The drawing under review shows one solid part. Ordinate dimensions are in mm from its lowest x, y, z. Coordinates: 2 decimals unless noted, no trailing zeros. Order: outer loops, then holes, each group sorted by start corner. A loop starts at its lowest first (then second) coordinate and runs counter-clockwise, first axis right, second up. Notation, with made-up numbers: M 46,46 L 82,46 A6 cw 82,53 Z; hole C 50,-4 d11. An arc over 180 degrees is marked long. Answer as a JSON object with one key per item and string values.
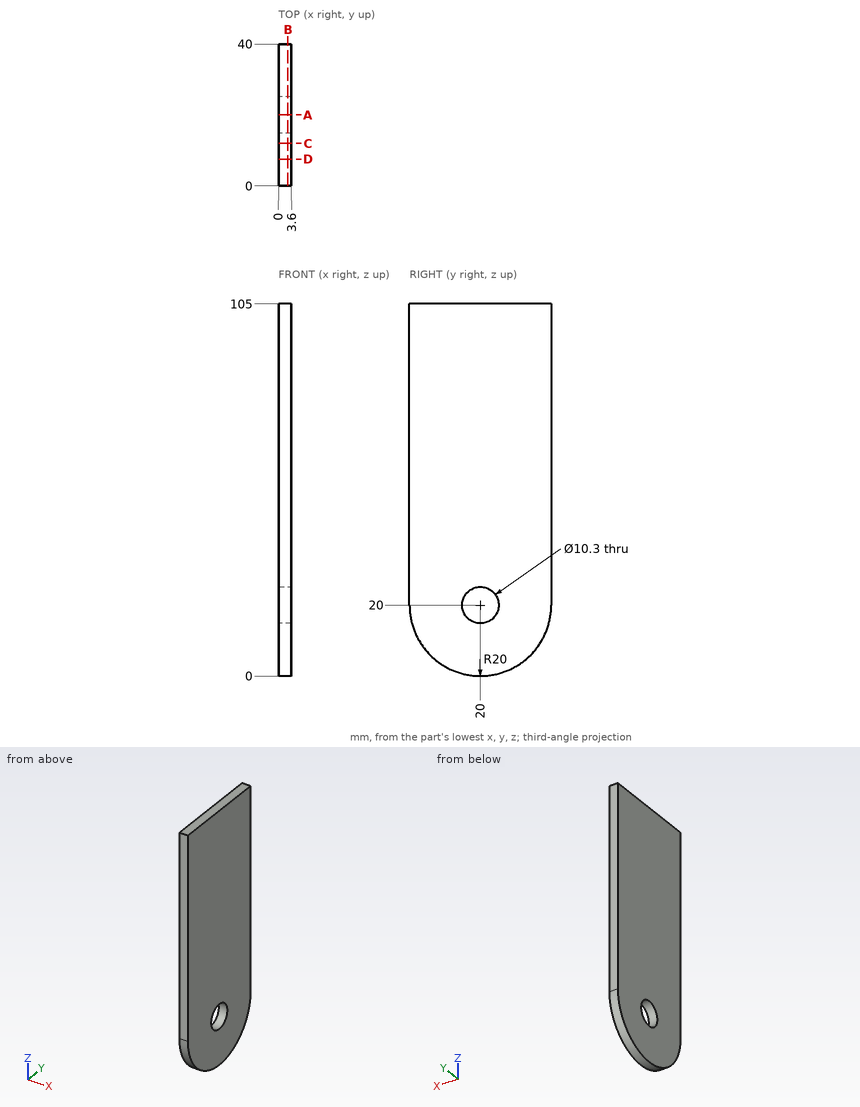
1) Add section C-C (y = 12). State the section outline as (x, z) points.
Taken from the geometry:
{"outline": "M 0,1.67 L 3.6,1.67 L 3.6,105 L 0,105 Z"}
2) Add section A-A (y = 20). State the section outline as (x, z) points.
Taken from the geometry:
{"outline": "M 0,0 L 3.6,0 L 3.6,14.85 L 0,14.85 Z; M 0,25.15 L 3.6,25.15 L 3.6,105 L 0,105 Z"}
3) Insertion check: pin 1 Ø12 at (y, z) = (29.5, 80) entering from -X. The pin has a flat end and moves straight along its axis. Give the tip position at first contact, or say it passes through.
Taken from the geometry:
{"pin 1": "stops at x = 0"}
4) Add section D-D (y = 7.5). State the section outline as (x, z) points.
Taken from the geometry:
{"outline": "M 0,4.39 L 3.6,4.39 L 3.6,105 L 0,105 Z"}
5) Add section B-B (x = 2.6). State the section outline as (y, z) points.
Taken from the geometry:
{"outline": "M 0,20 A20 ccw 40,20 L 40,105 L 0,105 Z; hole C 20,20 d10.3"}
6) To check wall thickness, follow L1, parallel to Y at x = 0.9, z = 20; L2, parallel to Z at x = 3.3, y = 23; L3, parallel to Z at x = 2.5, y = 22. State the ranges of each line that lie inside material, in increasing order.
Taken from the geometry:
{"L1": "y = 0 to 14.85, 25.15 to 40", "L2": "z = 0.23 to 15.81, 24.19 to 105", "L3": "z = 0.1 to 15.25, 24.75 to 105"}
